Here's how the part is built. I have some questions about the finished solid (model axes, mm). Give positions to 0.01 mm unless a question says otherwise; leave off trailing zeros. Loops run counter-clockwise (first coordinate to the right, second up) from the corner with the lowest first, then second, coordinate; pieces in that order, holes last.
Q1. If we section it at B-B (x = -7.5): Please give me the cut outline in (y, z), plus the area to 3 significant figures.
Q2. If we section it at C-C (y = -0.9): Give the number of separate pieces and of enclosed holes in the cut face, plus the area to 3 significant figures.
Q3. I need wall thicknesses on line 1 (Z direction, x = 17.65, y = -1.4); line 2 (Z direction, x = -25.15, y = -0.55); line 3 (X direction, y = -1.6, z = -15). Which ranges of each line are inside material? Lowest first, please.
Q4. If we section it at A-A (z = 6): Please give me the cut outline in (x, y), plus the area to 3 significant figures.
Q5. If we section it at D-D (z = -15.15): Please give me the cut outline in (x, y), plus the area to 3 significant figures.
from build123d import *

# Parameters (mm, degrees)
F0_W      = 75
F0_H      = 56
F1_DEPTH  = 2
F3_D      = 4.4
F5_D      = 3.3
F7_D      = 3.3
F8_W      = 47.5419834256
F8_H      = 19.9280381203
F9_DEPTH  = 25
F10_W     = 22.1011936665
F10_H     = 47.0907129347
F11_DEPTH = 25


with BuildPart() as f1:
    # F0 (on Front) → F1 (new body)
    with BuildSketch(Plane.XZ):
        Rectangle(F0_W, F0_H)
    extrude(amount=F1_DEPTH)

    # F3 (through all)
    with Locations(Plane.XZ.offset(2)):
        with Locations((-32.2, 0), (32.2, 0)):
            Hole(F3_D / 2)

    # F5 (through all)
    with Locations(Plane.XZ.offset(2)):
        with Locations((-25.15, 22.65), (-25.15, -22.65), (25.15, -22.65), (25.15, 22.65)):
            Hole(F5_D / 2)

    # F7 (through all)
    with Locations(Plane.XZ.offset(2)):
        with Locations((-17.65, 15.15), (-17.65, -15.15), (17.65, -15.15), (17.65, 15.15)):
            Hole(F7_D / 2)

    # F8 (on face) → F9 (cut)
    with BuildSketch(Plane.XZ.offset(2)):
        Rectangle(F8_W, F8_H)
    extrude(amount=-F9_DEPTH, mode=Mode.SUBTRACT)

    # F10 (on face) → F11 (cut)
    with BuildSketch(Plane.XZ.offset(2)):
        Rectangle(F10_W, F10_H)
    extrude(amount=-F11_DEPTH, mode=Mode.SUBTRACT)


solid = f1.part
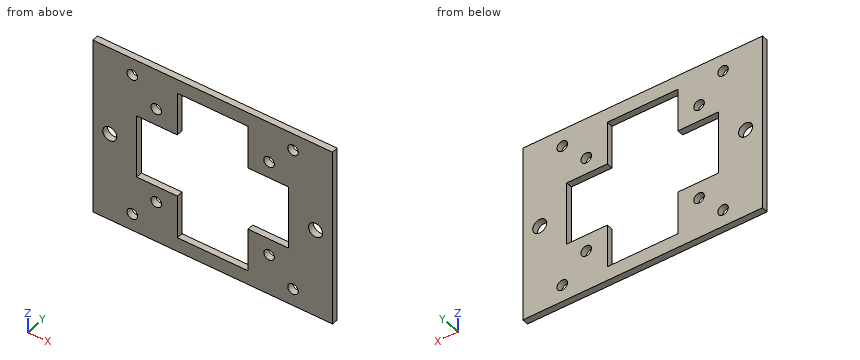
Check sheet entries:
1. outline: (-2, -28) - (0, -28) - (0, -23.55) - (-2, -23.55) - close; (-2, 23.55) - (0, 23.55) - (0, 28) - (-2, 28) - close
1. area: 17.8 mm2
2. separate pieces: 1
2. enclosed holes: 11
2. area: 2,550 mm2
3. line 1: z = -28 to -16.8, -13.5 to -9.96, 9.96 to 13.5, 16.8 to 28
3. line 2: z = -28 to -24.3, -21 to 21, 24.3 to 28
3. line 3: x = -37.5 to -19.29, -16.01 to -11.05, 11.05 to 16.01, 19.29 to 37.5
4. outline: (-37.5, -2) - (-23.77, -2) - (-23.77, 0) - (-37.5, 0) - close; (23.77, -2) - (37.5, -2) - (37.5, 0) - (23.77, 0) - close
4. area: 54.9 mm2
5. outline: (-37.5, -2) - (-19.3, -2) - (-19.3, 0) - (-37.5, 0) - close; (-16, -2) - (-11.05, -2) - (-11.05, 0) - (-16, 0) - close; (11.05, -2) - (16, -2) - (16, 0) - (11.05, 0) - close; (19.3, -2) - (37.5, -2) - (37.5, 0) - (19.3, 0) - close
5. area: 92.6 mm2
